Work out the finished part from the listing and answer in its coordinate system (mm). Round coordinates to 2 decimals unless told otherwise and drop trailing zeros. Order: outer loops, then holes, each group sorted by start corner. A loop starts at its lowest first (then second) coordinate and runs counter-clockwise, first axis right, second up. Notation, with made-up numbers: (34.25, 8) - (69.25, 8) arc R35 ccw to (69.25, 44) - close; hole circle Ø2 at (-39, 28). An arc over 180 degrees is marked (long way). Put each result on its own line as item: value.
```python
from build123d import *

# Parameters (mm, degrees)
SKETCH1_W           = 254
SKETCH1_H           = 177.8
BOSS_EXTRUDE1_DEPTH = 6.35
SKETCH2_W           = 25.4
SKETCH2_H           = 6.858
SKETCH2_W_2         = 6.858
SKETCH2_H_2         = 25.4
CUT_EXTRUDE1_DEPTH  = 156.15325488


with BuildPart() as part:
    # Sketch1 → Boss-Extrude1 (new body)
    with BuildSketch(Plane(origin=(0, 0, 0), x_dir=(1, 0, 0), z_dir=(0, 1, 0))):
        Rectangle(SKETCH1_W, SKETCH1_H)
    extrude(amount=BOSS_EXTRUDE1_DEPTH)

    # Sketch2 → Cut-Extrude1 (cut, through all)
    with BuildSketch(Plane(origin=(0, 0, 0), x_dir=(1, 0, 0), z_dir=(0, 1, 0))):
        with Locations((76.2, 66.675)):
            Rectangle(SKETCH2_W, SKETCH2_H)
        with Locations((-76.2, 66.675)):
            Rectangle(SKETCH2_W, SKETCH2_H)
        with BuildLine():
            Line((38.1, 85.979), (63.5, 85.979))
            ThreePointArc((63.5, 85.979), (66.929, 82.55), (63.5, 79.121))
            Line((63.5, 79.121), (38.1, 79.121))
            ThreePointArc((38.1, 79.121), (34.671, 82.55), (38.1, 85.979))
        make_face()
        with BuildLine():
            Line((88.9, 85.979), (114.3, 85.979))
            ThreePointArc((114.3, 85.979), (117.729, 82.55), (114.3, 79.121))
            Line((114.3, 79.121), (88.9, 79.121))
            ThreePointArc((88.9, 79.121), (85.471, 82.55), (88.9, 85.979))
        make_face()
        with BuildLine():
            Line((-114.3, 85.979), (-88.9, 85.979))
            ThreePointArc((-88.9, 85.979), (-85.471, 82.55), (-88.9, 79.121))
            Line((-88.9, 79.121), (-114.3, 79.121))
            ThreePointArc((-114.3, 79.121), (-117.729, 82.55), (-114.3, 85.979))
        make_face()
        with Locations((38.1, 66.675)):
            Rectangle(SKETCH2_W, SKETCH2_H)
        with BuildLine():
            Line((-63.5, 85.979), (-38.1, 85.979))
            ThreePointArc((-38.1, 85.979), (-34.671, 82.55), (-38.1, 79.121))
            Line((-38.1, 79.121), (-63.5, 79.121))
            ThreePointArc((-63.5, 79.121), (-66.929, 82.55), (-63.5, 85.979))
        make_face()
        with BuildLine():
            Line((-12.7, 85.979), (12.7, 85.979))
            ThreePointArc((12.7, 85.979), (16.129, 82.55), (12.7, 79.121))
            Line((12.7, 79.121), (-12.7, 79.121))
            ThreePointArc((-12.7, 79.121), (-16.129, 82.55), (-12.7, 85.979))
        make_face()
        with Locations((-104.775, 38.1)):
            Rectangle(SKETCH2_W_2, SKETCH2_H_2)
        with Locations((-104.775, 0)):
            Rectangle(SKETCH2_W_2, SKETCH2_H_2)
        with Locations((0, 66.675)):
            Rectangle(SKETCH2_W, SKETCH2_H)
        with Locations((-38.1, 66.675)):
            Rectangle(SKETCH2_W, SKETCH2_H)
        with BuildLine():
            Line((-124.079, -12.7), (-124.079, 12.7))
            ThreePointArc((-124.079, 12.7), (-120.65, 16.129), (-117.221, 12.7))
            Line((-117.221, 12.7), (-117.221, -12.7))
            ThreePointArc((-117.221, -12.7), (-120.65, -16.129), (-124.079, -12.7))
        make_face()
        with Locations((-104.775, -38.1)):
            Rectangle(SKETCH2_W_2, SKETCH2_H_2)
        with BuildLine():
            Line((-124.079, 38.1), (-124.079, 63.5))
            ThreePointArc((-124.079, 63.5), (-120.65, 66.929), (-117.221, 63.5))
            Line((-117.221, 63.5), (-117.221, 38.1))
            ThreePointArc((-117.221, 38.1), (-120.65, 34.671), (-124.079, 38.1))
        make_face()
        with BuildLine():
            Line((-124.079, -63.5), (-124.079, -38.1))
            ThreePointArc((-124.079, -38.1), (-120.65, -34.671), (-117.221, -38.1))
            Line((-117.221, -38.1), (-117.221, -63.5))
            ThreePointArc((-117.221, -63.5), (-120.65, -66.929), (-124.079, -63.5))
        make_face()
        with BuildLine():
            Line((124.079, -12.7), (124.079, 12.7))
            ThreePointArc((124.079, 12.7), (120.65, 16.129), (117.221, 12.7))
            Line((117.221, 12.7), (117.221, -12.7))
            ThreePointArc((117.221, -12.7), (120.65, -16.129), (124.079, -12.7))
        make_face()
        with BuildLine():
            Line((124.079, 38.1), (124.079, 63.5))
            ThreePointArc((124.079, 63.5), (120.65, 66.929), (117.221, 63.5))
            Line((117.221, 63.5), (117.221, 38.1))
            ThreePointArc((117.221, 38.1), (120.65, 34.671), (124.079, 38.1))
        make_face()
        with BuildLine():
            Line((124.079, -63.5), (124.079, -38.1))
            ThreePointArc((124.079, -38.1), (120.65, -34.671), (117.221, -38.1))
            Line((117.221, -38.1), (117.221, -63.5))
            ThreePointArc((117.221, -63.5), (120.65, -66.929), (124.079, -63.5))
        make_face()
        with Locations((104.775, -38.1)):
            Rectangle(SKETCH2_W_2, SKETCH2_H_2)
        with Locations((104.775, 38.1)):
            Rectangle(SKETCH2_W_2, SKETCH2_H_2)
        with Locations((104.775, 0)):
            Rectangle(SKETCH2_W_2, SKETCH2_H_2)
        with Locations((-38.1, -66.675)):
            Rectangle(SKETCH2_W, SKETCH2_H)
        with Locations((38.1, -66.675)):
            Rectangle(SKETCH2_W, SKETCH2_H)
        with Locations((0, -66.675)):
            Rectangle(SKETCH2_W, SKETCH2_H)
        with BuildLine():
            Line((12.7, -79.121), (-12.7, -79.121))
            ThreePointArc((-12.7, -79.121), (-16.129, -82.55), (-12.7, -85.979))
            Line((-12.7, -85.979), (12.7, -85.979))
            ThreePointArc((12.7, -85.979), (16.129, -82.55), (12.7, -79.121))
        make_face()
        with BuildLine():
            Line((-38.1, -79.121), (-63.5, -79.121))
            ThreePointArc((-63.5, -79.121), (-66.929, -82.55), (-63.5, -85.979))
            Line((-63.5, -85.979), (-38.1, -85.979))
            ThreePointArc((-38.1, -85.979), (-34.671, -82.55), (-38.1, -79.121))
        make_face()
        with BuildLine():
            Line((-88.9, -79.121), (-114.3, -79.121))
            ThreePointArc((-114.3, -79.121), (-117.729, -82.55), (-114.3, -85.979))
            Line((-114.3, -85.979), (-88.9, -85.979))
            ThreePointArc((-88.9, -85.979), (-85.471, -82.55), (-88.9, -79.121))
        make_face()
        with BuildLine():
            Line((114.3, -79.121), (88.9, -79.121))
            ThreePointArc((88.9, -79.121), (85.471, -82.55), (88.9, -85.979))
            Line((88.9, -85.979), (114.3, -85.979))
            ThreePointArc((114.3, -85.979), (117.729, -82.55), (114.3, -79.121))
        make_face()
        with BuildLine():
            Line((63.5, -79.121), (38.1, -79.121))
            ThreePointArc((38.1, -79.121), (34.671, -82.55), (38.1, -85.979))
            Line((38.1, -85.979), (63.5, -85.979))
            ThreePointArc((63.5, -85.979), (66.929, -82.55), (63.5, -79.121))
        make_face()
        with Locations((-76.2, -66.675)):
            Rectangle(SKETCH2_W, SKETCH2_H)
        with Locations((76.2, -66.675)):
            Rectangle(SKETCH2_W, SKETCH2_H)
    extrude(amount=CUT_EXTRUDE1_DEPTH, mode=Mode.SUBTRACT)


solid = part.part
```
1) Given pin 1 Ø3 at (x, z) = (89, -23) entering from -Y, flat-ended and moving along its own axis, determine where the tip first touches the part or whether it passes through.
Findings below:
pin 1: stops at y = 0
2) A cutting plane is placed at D-D on x = 72.5. Write down the section's boundary in (y, z).
Findings below:
outline: (0, -88.9) - (6.35, -88.9) - (6.35, -70.1) - (0, -70.1) - close; (0, -63.25) - (6.35, -63.25) - (6.35, 63.25) - (0, 63.25) - close; (0, 70.1) - (6.35, 70.1) - (6.35, 88.9) - (0, 88.9) - close
3) A cutting plane is placed at A-A on z = -43. Write down the section's boundary in (x, y), then the cut area to 3 significant figures.
Findings below:
outline: (-127, 0) - (-124.08, 0) - (-124.08, 6.35) - (-127, 6.35) - close; (-117.22, 0) - (-108.2, 0) - (-108.2, 6.35) - (-117.22, 6.35) - close; (-101.35, 0) - (101.35, 0) - (101.35, 6.35) - (-101.35, 6.35) - close; (108.2, 0) - (117.22, 0) - (117.22, 6.35) - (108.2, 6.35) - close; (124.08, 0) - (127, 0) - (127, 6.35) - (124.08, 6.35) - close
area: 1,440 mm2
4) A cutting plane is placed at B-B on x = -46.5. Write down the section's boundary in (y, z), then the cut area to 3 significant figures.
Findings below:
outline: (0, -88.9) - (6.35, -88.9) - (6.35, -85.98) - (0, -85.98) - close; (0, -79.12) - (6.35, -79.12) - (6.35, -70.1) - (0, -70.1) - close; (0, -63.25) - (6.35, -63.25) - (6.35, 63.25) - (0, 63.25) - close; (0, 70.1) - (6.35, 70.1) - (6.35, 79.12) - (0, 79.12) - close; (0, 85.98) - (6.35, 85.98) - (6.35, 88.9) - (0, 88.9) - close
area: 955 mm2
5) For a pull along Z with two mould halves and no side action, classify faces 1 (the flat face through (-105, 3, 12.7)), 2 (the flat face through (50.8, 3, 67)), 3 (the flat face through (127, 3, 1)), 4 (the flat face through (-2, 3, 88.9)) as pulls with the +Z half, pulls with the -Z half, needs draft (parallel to the pull), parting line crosses it, or undercut.
Findings below:
face 1: undercut
face 2: undercut
face 3: needs draft
face 4: pulls with the +Z half
6) A cutting plane is placed at C-C on z = 82.55. Write down the section's boundary in (x, y).
Findings below:
outline: (-127, 0) - (-117.73, 0) - (-117.73, 6.35) - (-127, 6.35) - close; (-85.47, 0) - (-66.93, 0) - (-66.93, 6.35) - (-85.47, 6.35) - close; (-34.67, 0) - (-16.13, 0) - (-16.13, 6.35) - (-34.67, 6.35) - close; (16.13, 0) - (34.67, 0) - (34.67, 6.35) - (16.13, 6.35) - close; (66.93, 0) - (85.47, 0) - (85.47, 6.35) - (66.93, 6.35) - close; (117.73, 0) - (127, 0) - (127, 6.35) - (117.73, 6.35) - close
7) Straight lines are drawn through the part: L1, parallel to X at y = 1.5, z = -49; L2, parallel to Z at x = 72, y = 5; L3, parallel to X at y = 3.5, z = -55.5. For each, find the intervals that lie inside material, in ascending order. Write a range as from..to.
Findings below:
L1: x = -127..-124.08, -117.22..-108.2, -101.35..101.35, 108.2..117.22, 124.08..127
L2: z = -88.9..-70.1, -63.25..63.25, 70.1..88.9
L3: x = -127..-124.08, -117.22..117.22, 124.08..127
